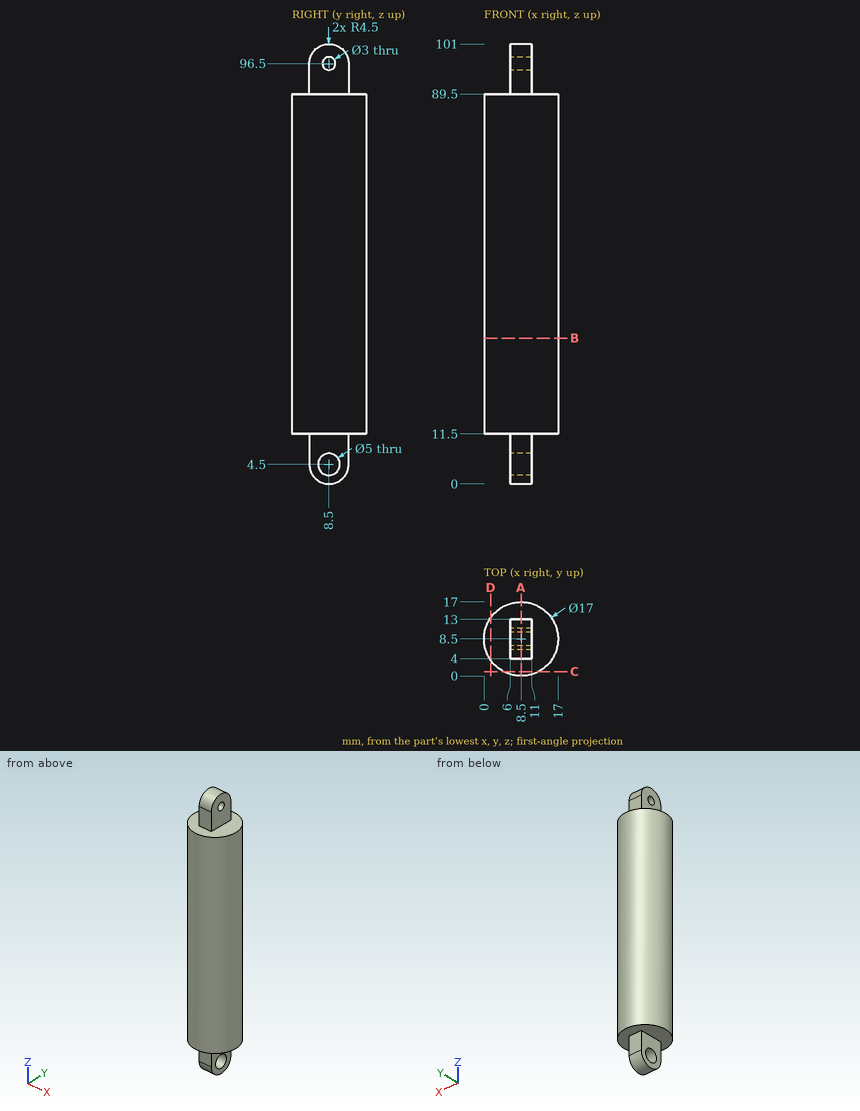
For this review, use the dimensioned drawing (mm, ordinates from the lowest corner) and the shaded views. Coordinates: 2 decimals unless noted, no trailing zeros. Write each loop counter-clockwise with the first axis right and the second up, starting at its lowest first coordinate (ties: lowest second). Pieces come first, ordered by that corner, then holes. Notation, with made-up numbers: (58.5, 85.25) -> (71.5, 85.25) arc R23 ccw to (71.5, 119.25) -> close; hole circle Ø11 at (-4.5, -8). An arc over 180 degrees is marked (long way). Put each result on its own line as item: value.
Q1. Wall thickness on L1, parallel to Y at x = 9.8, z = 96.5; L2, parallel to Z at x = 6.25, y = 9.5; L3, parallel to Y at x = 9.75, z = 4.5: over which ranges is each line inside the solid? List them lowest first.
From the geometry:
L1: y = 4 to 7, 10 to 13
L2: z = 0.11 to 2.21, 6.79 to 95.38, 97.62 to 100.89
L3: y = 4 to 6, 11 to 13
Q2. Take a section at C-C, the plane y = 1. State the section outline as (x, z) points.
From the geometry:
outline: (4.5, 11.5) -> (12.5, 11.5) -> (12.5, 89.5) -> (4.5, 89.5) -> close
Q3. Take a section at A-A, the plane x = 8.5. State the section outline as (y, z) points, then the cut area to 3 significant figures.
From the geometry:
outline: (0, 11.5) -> (4, 11.5) -> (4, 4.5) arc R4.5 ccw to (13, 4.5) -> (13, 11.5) -> (17, 11.5) -> (17, 89.5) -> (13, 89.5) -> (13, 96.5) arc R4.5 ccw to (4, 96.5) -> (4, 89.5) -> (0, 89.5) -> close; hole circle Ø5 at (8.5, 4.5); hole circle Ø3 at (8.5, 96.5)
area: 1,490 mm2
Q4. Clearance check with flat-ended pins moving along their axes: pin 1 Ø7 at (y, z) = (10.5, 7) entering from -X; pin 2 Ø1.5 at (x, z) = (8.5, 94) entering from +Y; pin 3 Ø2.5 at (y, z) = (9, 97.5) entering from +X; pin 4 Ø3 at (y, z) = (8.5, 4.5) entering from +X. State where each tip first meets the part, or that it passes through.
From the geometry:
pin 1: stops at x = 6
pin 2: stops at y = 13
pin 3: stops at x = 11
pin 4: passes through
Q5. Take a section at D-D, the plane x = 1.5. State the section outline as (y, z) points, then the cut area to 3 significant figures.
From the geometry:
outline: (3.68, 11.5) -> (13.32, 11.5) -> (13.32, 89.5) -> (3.68, 89.5) -> close
area: 752 mm2
Q6. Take a section at B-B, the plane z = 33.5. State the section outline as (x, y) points, then the cut area to 3 significant figures.
From the geometry:
outline: circle Ø17 at (8.5, 8.5)
area: 227 mm2
